The listing builds one solid part. Answer for the finished solid, in the listing's coordinates (mm). Round coordinates to 2 decimals unless told otherwise and drop trailing zeros. Write each loop counter-clockwise with the first axis right and the second up, starting at its lowest first coordinate (ties: lowest second). Pieces come first, ordered by that corner, then holes.
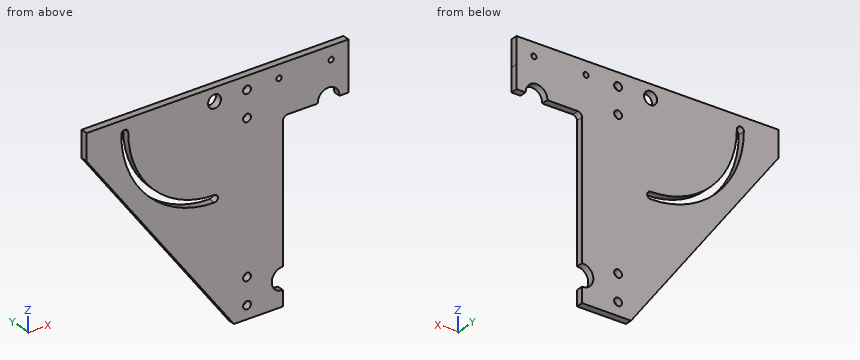
from build123d import *

# Parameters (mm, degrees)
F2_DEPTH = 8
F4_D     = 15
F6_D     = 9
F8_DEPTH = 25
F9_D     = 6


with BuildPart() as f2:
    # F1 (on Front) → F2 (new body)
    with BuildSketch(Plane.XZ):
        with BuildLine():
            Line((-257.7572688935, 147.7572688894), (-257.7572688935, 117.7572688894))
            Line((-257.7572688935, 117.7572688894), (-87.7572688935, -111.2427311235))
            Line((-87.7572688935, -111.2427311235), (-57.7572688935, -111.2427311235))
            Line((-57.7572688935, -111.2427311235), (-31.2572688938, -111.2427311235))
            Line((-31.2572688938, -111.2427311235), (-31.2572688938, -93.7327271198))
            ThreePointArc((-31.2572688938, -93.7327271198), (-44.2572688934, -81.2427311229), (-31.2572688938, -68.7527351261))
            Line((-31.2572688938, -68.7527351261), (-31.2572688938, 86.2572688893))
            ThreePointArc((-31.2572688938, 86.2572688893), (-29.7928027997, 89.7928027952), (-26.2572688938, 91.2572688893))
            Line((-26.2572688938, 91.2572688893), (8.7527351631, 91.2572688893))
            ThreePointArc((8.7527351631, 91.2572688893), (21.2427311599, 104.2572688889), (33.7327271567, 91.2572688893))
            Line((33.7327271567, 91.2572688893), (44.2427311605, 91.2572688893))
            Line((44.2427311605, 91.2572688893), (44.2427311606, 117.757268889))
            Line((44.2427311606, 117.757268889), (44.2427311606, 147.7572688894))
            Line((44.2427311606, 147.7572688894), (-257.7572688935, 147.7572688894))
        make_face()
    extrude(amount=-F2_DEPTH)

    # F4 (through all)
    with Locations(Plane.XZ):
        with Locations((-110.2572688394, 132.7572688894)):
            Hole(F4_D / 2)

    # F6 (through all)
    with Locations(Plane.XZ):
        with Locations((-72.7572688936, -66.2427311235), (-72.7572688936, -96.2427311235), (-72.7572688936, 132.7572688894), (-72.7572688936, 102.7572688894)):
            Hole(F6_D / 2)

    # F7 (on face) → F8 (cut)
    with BuildSketch(Plane.XZ):
        with BuildLine():
            ThreePointArc((-110.2705276792, 33.2572697728), (-180.6190811191, 62.4048320253), (-209.7572688394, 132.7572688894))
            ThreePointArc((-209.7572688394, 132.7572688894), (-213.7572688394, 136.7572688894), (-217.7572688394, 132.7572688894))
            ThreePointArc((-217.7572688394, 132.7572688894), (-186.2763122571, 56.7483546894), (-110.2715937166, 25.2572698438))
            ThreePointArc((-110.2715937166, 25.2572698438), (-106.2710607334, 29.2567367896), (-110.2705276792, 33.2572697728))
        make_face()
    extrude(amount=-F8_DEPTH, mode=Mode.SUBTRACT)

    # F9 (through all)
    with Locations(Plane.XZ):
        with Locations((-35.7572688394, 132.7572688894), (24.2427311606, 132.7572688894)):
            Hole(F9_D / 2)


solid = f2.part
1. Given pin 1 (1.5 mm diameter, centred on y = 1.5, z = 6, fed in from +X); pin 2 (1 mm diameter, centred on y = 1.5, z = 0.5, fed in from -X); pin 3 (2.5 mm diameter, centred on x = 37, y = 2, fed in from -Z), each flat-ended and moving along its own axis, determine where each tip first touches the part or whether it passes through.
Geometry says:
pin 1: stops at x = -31.26
pin 2: stops at x = -171.08
pin 3: stops at z = 91.26
2. Straight lines are drawn through the part: line 1 along Z through (x, y) = (-72.5, 1.25); line 2 along X through (y, z) = (5, 132); line 3 along X through (y, z) = (1.25, 92). For each, find the intervals that lie inside material, in ascending order.
Geometry says:
line 1: z = -111.24 to -100.74, -91.75 to -70.74, -61.75 to 98.26, 107.25 to 128.26, 137.25 to 147.76
line 2: x = -257.76 to -217.75, -209.75 to -117.72, -102.8 to -77.19, -68.32 to -38.66, -32.85 to 21.34, 27.15 to 44.24
line 3: x = -238.64 to -209.73, -201.03 to 8.75, 33.74 to 44.24
3. Section C-C on y = 2.75 is taken. Give the number of separate pieces and of enclosed holes in the cut face, plus the area to 3 significant figures.
Geometry says:
separate pieces: 1
enclosed holes: 8
area: 41,100 mm2
4. Section A-A on z = 113.5 is taken. Determine the outline of the cut face in (x, y).
Geometry says:
outline: (-254.6, 0) - (-216.02, 0) - (-216.02, 8) - (-254.6, 8) - close; (-207.88, 0) - (44.24, 0) - (44.24, 8) - (-207.88, 8) - close
5. Section D-D on x = -18 is taken. Determine the outline of the cut face in (y, z), plus the area to 3 significant figures.
Geometry says:
outline: (0, 91.26) - (8, 91.26) - (8, 147.76) - (0, 147.76) - close
area: 452 mm2
6. Section B-B on x = -129.5 is taken. Determine the outline of the cut face in (y, z), plus the area to 3 significant figures.
Geometry says:
outline: (0, -55.01) - (8, -55.01) - (8, 26.99) - (0, 26.99) - close; (0, 35.14) - (8, 35.14) - (8, 147.76) - (0, 147.76) - close
area: 1,560 mm2
